The listing builds one solid part. Answer for the finished solid, in the listing's coordinates (mm). Coordinates: 2 decimals unless noted, no trailing zeros. Loops run counter-clockwise (first coordinate to the right, second up) from the corner with the lowest first, then second, coordinate; pieces in that order, holes last. Notation, with made-up numbers: M -20,16 L 15,16 A24 ccw 15,34 Z; hole C -20,-33 d11. An arc over 180 degrees is marked long. Answer as a JSON object with one key per item and string values. Group by question number.
1. A cutting plane is placed at D-D on x = -31.5. Give the vertices of the cut face in (y, z).
2. A cutting plane is placed at C-C on y = 1.5. Give the vertices of the cut face in (x, z), and give its area (3 significant figures).
3. A cutting plane is placed at B-B on z = 1. State how many separate pieces and enclosed holes the cut face has, and give its area (3 significant figures).
4. A cutting plane is placed at A-A on y = 21. Give the vertices of the cut face in (x, z), and give its area (3 significant figures).
5. Straight lines are drawn through the part: L1, parallel to X at y = 15, z = 3.25; L2, parallel to X at y = 31, z = 3.75; L3, parallel to X at y = 34, z = 4.75. For each, find the intervals that lie inside material, in ascending order.
6. Given pin 1 (3 mm diameter, centred on x = 51, z = 1.5, fed in from +Y); pin 2 (3 mm diameter, centred on y = 37, z = 4.5, fed in from -X); pin 3 (3 mm diameter, centred on y = 2.5, z = 4.5, fed in from +X); pin 4 (1 mm diameter, centred on x = 42, y = 6.5, fed in from +Z), each flat-ended and moving along its own axis, determine where each tip first touches the part or whether it passes through.
from build123d import *

# Parameters (mm, degrees)
BOSS_EXTRUDE1_DEPTH = 6.4


with BuildPart() as part:
    # Sketch1 → Boss-Extrude1 (new body)
    with BuildSketch(Plane.XY):
        Polygon((30.862718171, 33.494054131), (69.862718171, 33.494054131), (69.862718171, 8.494054131), (30.862718171, 8.494054131), (30.862718171, -9.005945869), (-39.137281829, -9.005945869), (-39.137281829, 28.472304637), (-17.137281829, 28.472304637), (-17.137281829, 50.994054131), (30.862718171, 50.994054131), align=None)
        with BuildLine():
            Line((-4.137281829, 38.994054131), (-4.137281829, -1.005945869))
            ThreePointArc((-4.137281829, -1.005945869), (-1.637281829, -3.505945869), (0.862718171, -1.005945869))
            Line((0.862718171, -1.005945869), (0.862718171, 38.994054131))
            ThreePointArc((0.862718171, 38.994054131), (-1.637281829, 41.494054131), (-4.137281829, 38.994054131))
        make_face(mode=Mode.SUBTRACT)
        with BuildLine():
            Line((-12.137281829, 33.312431903), (-12.137281829, 2.809827896))
            ThreePointArc((-12.137281829, 2.809827896), (-9.637281829, 0.309827896), (-7.137281829, 2.809827896))
            Line((-7.137281829, 2.809827896), (-7.137281829, 33.312431903))
            ThreePointArc((-7.137281829, 33.312431903), (-9.637281829, 35.812431903), (-12.137281829, 33.312431903))
        make_face(mode=Mode.SUBTRACT)
        with BuildLine():
            Line((-15.137281829, 23.861283589), (-15.137281829, 7.683449462))
            ThreePointArc((-15.137281829, 7.683449462), (-17.637281829, 5.183449462), (-20.137281829, 7.683449462))
            Line((-20.137281829, 7.683449462), (-20.137281829, 23.861283589))
            ThreePointArc((-20.137281829, 23.861283589), (-17.637281829, 26.361283589), (-15.137281829, 23.861283589))
        make_face(mode=Mode.SUBTRACT)
        with BuildLine():
            Line((3.862718171, 30.994054131), (3.862718171, 2.647434443))
            ThreePointArc((3.862718171, 2.647434443), (6.362718171, 0.147434443), (8.862718171, 2.647434443))
            Line((8.862718171, 2.647434443), (8.862718171, 30.994054131))
            ThreePointArc((8.862718171, 30.994054131), (6.362718171, 33.494054131), (3.862718171, 30.994054131))
        make_face(mode=Mode.SUBTRACT)
        with BuildLine():
            Line((11.862718171, 22.048271006), (11.862718171, 5.538473012))
            ThreePointArc((11.862718171, 5.538473012), (14.362718171, 3.038473012), (16.862718171, 5.538473012))
            Line((16.862718171, 5.538473012), (16.862718171, 22.048271006))
            ThreePointArc((16.862718171, 22.048271006), (14.362718171, 24.548271006), (11.862718171, 22.048271006))
        make_face(mode=Mode.SUBTRACT)
    extrude(amount=BOSS_EXTRUDE1_DEPTH)


solid = part.part
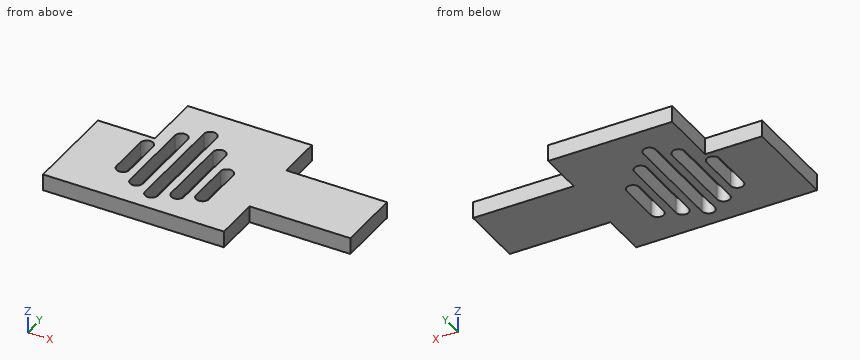
From the geometry:
{
 "1": {"outline": "M -9.01,0 L 28.47,0 L 28.47,6.4 L -9.01,6.4 Z"},
 "2": {"outline": "M -39.14,0 L -11.77,0 L -11.77,6.4 L -39.14,6.4 Z; M -7.51,0 L -4.14,0 L -4.14,6.4 L -7.51,6.4 Z; M 0.86,0 L 4.14,0 L 4.14,6.4 L 0.86,6.4 Z; M 8.58,0 L 30.86,0 L 30.86,6.4 L 8.58,6.4 Z", "area": "360 mm²"},
 "3": {"separate pieces": "1", "enclosed holes": "5", "area": "3,920 mm²"},
 "4": {"outline": "M -39.14,0 L -20.14,0 L -20.14,6.4 L -39.14,6.4 Z; M -15.14,0 L -12.14,0 L -12.14,6.4 L -15.14,6.4 Z; M -7.14,0 L -4.14,0 L -4.14,6.4 L -7.14,6.4 Z; M 0.86,0 L 3.86,0 L 3.86,6.4 L 0.86,6.4 Z; M 8.86,0 L 11.86,0 L 11.86,6.4 L 8.86,6.4 Z; M 16.86,0 L 69.86,0 L 69.86,6.4 L 16.86,6.4 Z", "area": "538 mm²"},
 "5": {"L1": "x = -39.14 to -20.14, -15.14 to -12.14, -7.14 to -4.14, 0.86 to 3.86, 8.86 to 11.86, 16.86 to 69.86", "L2": "x = -17.14 to -12.14, -7.14 to -4.14, 0.86 to 3.86, 8.86 to 69.86", "L3": "x = -17.14 to -12.04, -7.23 to -4.14, 0.86 to 30.86"},
 "6": {"pin 1": "stops at y = 33.49", "pin 2": "stops at x = -17.14", "pin 3": "stops at x = 30.86", "pin 4": "passes through"}
}
